Geometry check sheet. Reference: the model listing, model coordinates, mm. Round coordinates to 2 decimals unless told otherwise and drop trailing zeros. Order: outer loops, then holes, each group sorted by start corner. A loop starts at its lowest first (then second) coordinate and runs counter-clockwise, first axis right, second up.
```python
from build123d import *

# Parameters (mm, degrees)
BOSS_EXTRUDE2_DEPTH = 6.3
SKETCH1_7_R         = 2.55
CUT_EXTRUDE3_DEPTH  = 141.148813766
SKETCH1_8_R         = 3.65
CUT_EXTRUDE4_DEPTH  = 141.148813766
SKETCH1_9_R         = 2.55
CUT_EXTRUDE5_DEPTH  = 141.148813766
SKETCH1_10_R        = 3.65
CUT_EXTRUDE6_DEPTH  = 141.148813766
SKETCH1_11_R        = 2.05
CUT_EXTRUDE8_DEPTH  = 141.148813766
SKETCH1_12_R        = 2.05
CUT_EXTRUDE10_DEPTH = 141.148813766
SKETCH1_13_R        = 2.55
CUT_EXTRUDE11_DEPTH = 141.148813766
SKETCH1_14_R        = 2.05
CUT_EXTRUDE12_DEPTH = 141.148813766
SKETCH1_15_R        = 2.05
CUT_EXTRUDE13_DEPTH = 141.148813766
SKETCH1_16_R        = 2.55
CUT_EXTRUDE14_DEPTH = 141.148813766
FILLET1_R           = 5
FILLET2_R           = 5
FILLET3_R           = 10
FILLET4_R           = 10
FILLET5_R           = 10


with BuildPart() as part:
    # Sketch1 → Boss-Extrude2 (new body)
    with BuildSketch(Plane(origin=(0, 0, 0), x_dir=(1, 0, 0), z_dir=(0, 1, 0))):
        Polygon((0, 64), (48, 64), (48, 99), (79, 99), (99, 64), (99, 0), (0, 0), align=None)
    extrude(amount=BOSS_EXTRUDE2_DEPTH)

    # Sketch1_7 → Cut-Extrude3 (cut, through all)
    with BuildSketch(Plane(origin=(0, 0, 0), x_dir=(1, 0, 0), z_dir=(0, 1, 0))):
        with Locations(Location((73.5, 89, 0), (0, 0, 270))):
            Circle(SKETCH1_7_R)
    extrude(amount=CUT_EXTRUDE3_DEPTH, mode=Mode.SUBTRACT)

    # Sketch1_8 → Cut-Extrude4 (cut, through all)
    with BuildSketch(Plane(origin=(0, 0, 0), x_dir=(1, 0, 0), z_dir=(0, 1, 0))):
        with Locations(Location((90, 54, 0), (0, 0, 270))):
            Circle(SKETCH1_8_R)
    extrude(amount=CUT_EXTRUDE4_DEPTH, mode=Mode.SUBTRACT)

    # Sketch1_9 → Cut-Extrude5 (cut, through all)
    with BuildSketch(Plane(origin=(0, 0, 0), x_dir=(1, 0, 0), z_dir=(0, 1, 0))):
        with Locations(Location((58, 73.5, 0), (0, 0, 270))):
            Circle(SKETCH1_9_R)
    extrude(amount=CUT_EXTRUDE5_DEPTH, mode=Mode.SUBTRACT)

    # Sketch1_10 → Cut-Extrude6 (cut, through all)
    with BuildSketch(Plane(origin=(0, 0, 0), x_dir=(1, 0, 0), z_dir=(0, 1, 0))):
        with Locations(Location((10, 54, 0), (0, 0, 270))):
            Circle(SKETCH1_10_R)
    extrude(amount=CUT_EXTRUDE6_DEPTH, mode=Mode.SUBTRACT)

    # Sketch1_11 → Cut-Extrude8 (cut, through all)
    with BuildSketch(Plane(origin=(0, 0, 0), x_dir=(1, 0, 0), z_dir=(0, 1, 0))):
        with Locations(Location((60, 49, 0), (0, 0, 270))):
            Circle(SKETCH1_11_R)
    extrude(amount=CUT_EXTRUDE8_DEPTH, mode=Mode.SUBTRACT)

    # Sketch1_12 → Cut-Extrude10 (cut, through all)
    with BuildSketch(Plane(origin=(0, 0, 0), x_dir=(1, 0, 0), z_dir=(0, 1, 0))):
        with Locations(Location((40, 49, 0), (0, 0, 270))):
            Circle(SKETCH1_12_R)
    extrude(amount=CUT_EXTRUDE10_DEPTH, mode=Mode.SUBTRACT)

    # Sketch1_13 → Cut-Extrude11 (cut, through all)
    with BuildSketch(Plane(origin=(0, 0, 0), x_dir=(1, 0, 0), z_dir=(0, 1, 0))):
        with Locations(Location((90, 10, 0), (0, 0, 270))):
            Circle(SKETCH1_13_R)
    extrude(amount=CUT_EXTRUDE11_DEPTH, mode=Mode.SUBTRACT)

    # Sketch1_14 → Cut-Extrude12 (cut, through all)
    with BuildSketch(Plane(origin=(0, 0, 0), x_dir=(1, 0, 0), z_dir=(0, 1, 0))):
        with Locations(Location((60, 15, 0), (0, 0, 270))):
            Circle(SKETCH1_14_R)
    extrude(amount=CUT_EXTRUDE12_DEPTH, mode=Mode.SUBTRACT)

    # Sketch1_15 → Cut-Extrude13 (cut, through all)
    with BuildSketch(Plane(origin=(0, 0, 0), x_dir=(1, 0, 0), z_dir=(0, 1, 0))):
        with Locations(Location((40, 15, 0), (0, 0, 270))):
            Circle(SKETCH1_15_R)
    extrude(amount=CUT_EXTRUDE13_DEPTH, mode=Mode.SUBTRACT)

    # Sketch1_16 → Cut-Extrude14 (cut, through all)
    with BuildSketch(Plane(origin=(0, 0, 0), x_dir=(1, 0, 0), z_dir=(0, 1, 0))):
        with Locations(Location((10, 10, 0), (0, 0, 270))):
            Circle(SKETCH1_16_R)
    extrude(amount=CUT_EXTRUDE14_DEPTH, mode=Mode.SUBTRACT)

    # Fillet1
    fillet1_edges = [part.edges().sort_by_distance(p)[0] for p in [
        (0, 3.15, 0),
        (0, 3.15, -64),
        (99, 3.15, 0),
    ]]
    fillet(fillet1_edges, radius=FILLET1_R)

    # Fillet2
    fillet2_edges = [part.edges().sort_by_distance(p)[0] for p in [
        (79, 3.15, -99),
    ]]
    fillet(fillet2_edges, radius=FILLET2_R)

    # Fillet3
    fillet3_edges = [part.edges().sort_by_distance(p)[0] for p in [
        (48, 3.15, -99),
    ]]
    fillet(fillet3_edges, radius=FILLET3_R)

    # Fillet4
    fillet4_edges = [part.edges().sort_by_distance(p)[0] for p in [
        (99, 3.15, -64),
    ]]
    fillet(fillet4_edges, radius=FILLET4_R)

    # Fillet5
    fillet5_edges = [part.edges().sort_by_distance(p)[0] for p in [
        (48, 3.15, -64),
    ]]
    fillet(fillet5_edges, radius=FILLET5_R)


solid = part.part
```
(1) Sectioned sample at D-D, the plane x = 51. Record the cut outline in (y, z).
Returned:
outline: (0, -96.14) - (6.3, -96.14) - (6.3, 0) - (0, 0) - close
(2) Sectioned sample at A-A, the plane x = 10. Record the cut outline in (y, z), and give its area (3 significant figures).
Returned:
outline: (0, -64) - (6.3, -64) - (6.3, -57.65) - (0, -57.65) - close; (0, -50.35) - (6.3, -50.35) - (6.3, -12.55) - (0, -12.55) - close; (0, -7.45) - (6.3, -7.45) - (6.3, 0) - (0, 0) - close
area: 325 mm2
(3) Material ranges on line 1 (X direction, y = 3.5, z = -10); line 2 (X direction, y = 3, z = -54); line 3 (Z direction, x = 40, y = 2.25), recorded low to high.
Returned:
line 1: x = 0 to 7.45, 12.55 to 87.45, 92.55 to 99
line 2: x = 0 to 6.35, 13.65 to 86.35, 93.65 to 99
line 3: z = -64.2 to -51.05, -46.95 to -17.05, -12.95 to 0
(4) Depth check by flat-ended pin: P1, Ø6, axis at x = 58, z = -73.5, coming from the +Y side; P2, Ø1.9, axis at x = 16.5, y = 2.5, coming from the -Z side; P3, Ø3, axis at y = 2.5, z = -79.5, coming from the -X side. Enter the tip coordinate at first touch or a pass-through.
Returned:
P1: stops at y = 6.3
P2: stops at z = -64
P3: stops at x = 48
(5) Sectioned sample at B-B, the plane z = -55.5. Record the cut outline in (x, y).
Returned:
outline: (0, 0) - (6.67, 0) - (6.67, 6.3) - (0, 6.3) - close; (13.33, 0) - (86.67, 0) - (86.67, 6.3) - (13.33, 6.3) - close; (93.33, 0) - (99, 0) - (99, 6.3) - (93.33, 6.3) - close
(6) Sectioned sample at C-C, the plane y = 2.5. Give the number of separate pieces and of enclosed holes in the cut face, and give its area (3 significant figures).
Returned:
separate pieces: 1
enclosed holes: 10
area: 7,530 mm2
(7) Draft check along Z on faces 1 (the cylindrical face through (7.51, 3.11, -10.55)), 2 (the cylindrical face through (62.033, 3.106, -15.267)), 3 (the flat face through (67, 3, -99)), 4 (the flat face through (48, 3, -81)). Enter one of: released by +Z, released by -Z, zero draft, split by the parting line, or undercut.
Returned:
face 1: undercut
face 2: undercut
face 3: released by -Z
face 4: zero draft
